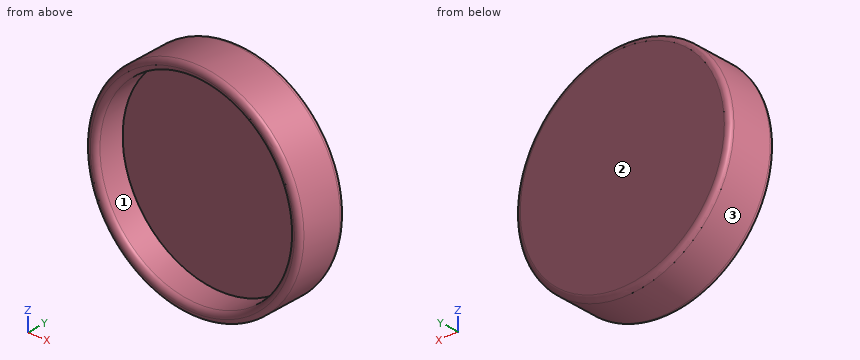
Autodesk Inventor part; units mm, degrees
ref_plane "YZ Plane" through (0, 0, 0) normal (1, 0, 0) x (0, 1, 0)
ref_plane "XZ Plane" through (0, 0, 0) normal (0, 1, 0) x (-1, 0, 0)
ref_plane "XY Plane" through (0, 0, 0) normal (0, 0, 1) x (1, 0, 0)
sketch "Sketch1" plane through (0, 0, 0) normal (0, 1, 0) x (-1, 0, 0)
  circle A0 centre (0, 0) radius 9.5
  circle A1 centre (0, 0) radius 10.5
  dimension "d0" = 19
  dimension "d1" = 21
extrude "Extrusion1" add sketch "Sketch1" along normal blind 5 contours A0 | A1
sketch "Sketch2" plane through (0, 0, 0) normal (0, -1, 0) x (1, 0, 0)
  circle A0 centre (0, 0) radius 9.5
  dimension "d4" = 19
extrude "Extrusion2" cut sketch "Sketch2" against normal blind 3
fillet "Fillet1" radius 0.5 1 edges at (10.5, 5, 0)
fillet "Fillet2" radius 0.5 2 edges at (-9.5, 0, 0) (10.5, 0, 0)
properties part number "Tapa Mirilla" material "LCP Plastic"
Build history of the part. All positions in model axes, mm. Face numbers are marked on the shaded views. Round coordinates to 2 decimals unless told otherwise and drop trailing zeros. Loops run counter-clockwise (first coordinate to the right, second up) from the corner with the lowest first, then second, coordinate; pieces in that order, holes last. Notation, with made-up numbers: M 81.25,10 L 123.25,10 A7 cw 123.25,22 Z; hole C 45.25,60 d8. An arc over 180 degrees is marked long. Answer as CSV lines item,"result".
1. Two-plate mould, pull along X, no slides. Class the marked faces 1, 2 and 3: released by +X, released by -X, zero draft, split by the parting line, or undercut.
Resolved:
face 1,"undercut"
face 2,"zero draft"
face 3,"split by the parting line"
2. Flat gauge pins, fed straight in: P1, Ø5.5, axis at x = -4.5, z = 0, coming from the -Y side; P2, Ø5, axis at x = -5, z = -6.5, coming from the -Y side; P3, Ø1, axis at y = 4, z = 7.5, coming from the -X side; P4, Ø3, axis at x = -2, y = 3, coming from the -Z side. Where does each tip first touch, or does it go through?
Resolved:
P1,"stops at y = 3"
P2,"stops at y = 0"
P3,"stops at x = -7.83"
P4,"stops at z = -10.49"
3. Wall check: probe 1 along Z at (x, y) = (0, 1.25); probe 2 along Y at (x, z) = (3.25, 2); probe 3 along Z at (x, y) = (-8, 1.45). Give the ranges that are in metal, low to high. Write a range as [from, to].
Resolved:
probe 1,"z = [-10.5, -9.5], [9.5, 10.5]"
probe 2,"y = [3, 5]"
probe 3,"z = [-6.8, -5.12], [5.12, 6.8]"
4. Cut at D-D on y = 4.15. Write the cut outline in (x, z).
Resolved:
outline,"C 0,0 d21"
5. Cut at C-C on y = 2.65. Write the cut outline in (x, z).
Resolved:
outline,"C 0,0 d21; hole C 0,0 d19"
